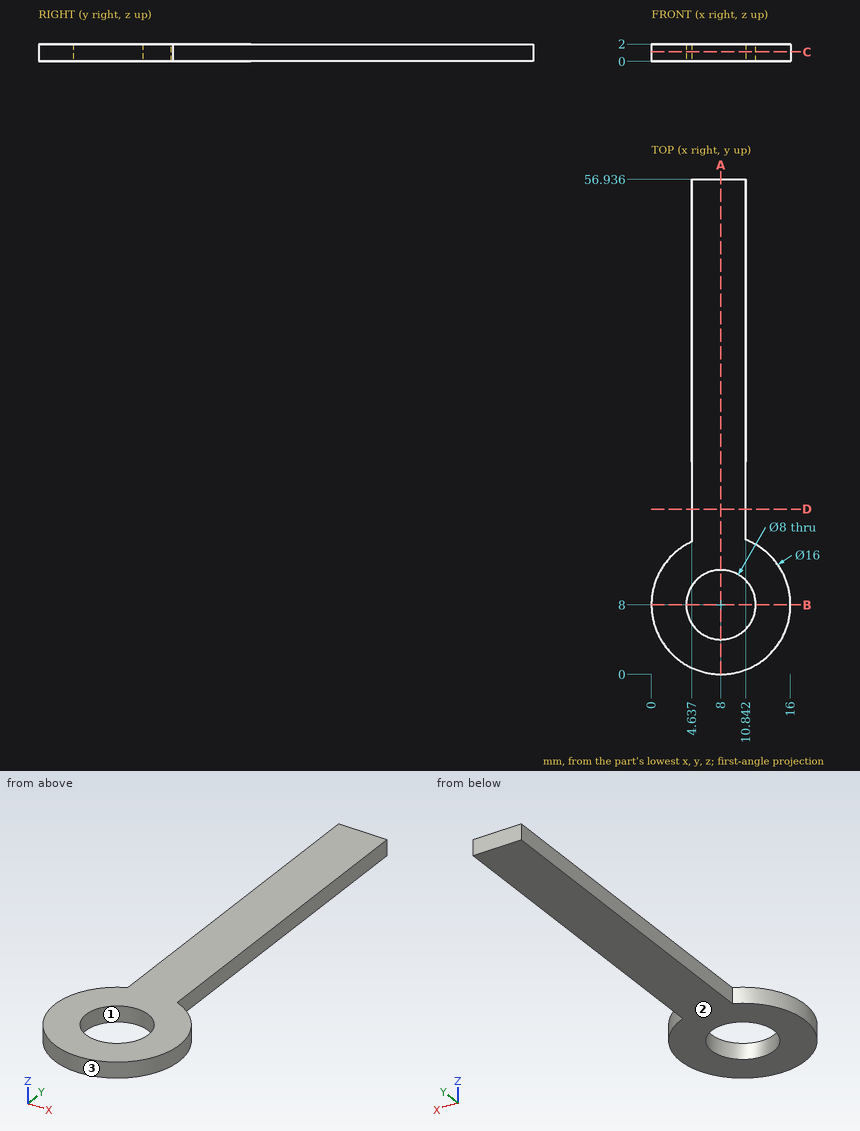
Drawing for the job (mm, zero at the part's lowest x, y, z). Give positions to 0.01 mm unless a question says otherwise; leave off trailing zeros. Order: outer loops, then holes, each group sorted by start corner. A loop starts at its lowest first (then second) coordinate and runs counter-clockwise, first axis right, second up. Notation, with made-up numbers: M 49,30.25 L 105,30.25 A13 cw 105,43.25 Z; hole C 52,-19 d1. An arc over 180 degrees is marked long. Use a Markdown table: item, result. Add a question column.
(1) Saw through at D-D, the plane y = 19. Give the cut face in (x, z).
(2) Drop a flat-ended pin along its axis: P1, Ø0.6, axis at y = 38, z = 1.5, coming from the +X side. Give the stop position or say it passes through.
(3) Saw through at B-B, the plane y = 8. Give the cut face in (x, z).
(4) Mould opens along Y. For the marked faces 1, 2 and 3 say: +Y half, -Y half, draft (parallel to the pull), parting line (faces both ways), or undercut.
(5) Probe line 1 along Y through (x, z) = (8, 1.05) (1 decimal); line 2 along X through (y, z) = (5, 1.3) (1 decimal); line 3 along X through (y, z) = (22, 0.55). List the from-to ranges inside material, lowest first. Write a range as [from, to].
(6) Saw through at C-C, the plane z = 1.1. Give the cut face in (x, y) (1 decimal).
(7) Saw through at A-A, the plane x = 8. Give the cut face in (y, z) (1 decimal).
Answer key:
| question | item | result |
|---|---|---|
| 1 | outline | M 4.64,0 L 10.84,0 L 10.84,2 L 4.64,2 Z |
| 2 | P1 | x = 10.84 |
| 3 | outline | M 0,0 L 4,0 L 4,2 L 0,2 Z; M 12,0 L 16,0 L 16,2 L 12,2 Z |
| 4 | face 1 | undercut |
| 4 | face 2 | draft |
| 4 | face 3 | parting line |
| 5 | line 1 | [0, 4], [12, 56.9] |
| 5 | line 2 | [0.6, 5.4], [10.6, 15.4] |
| 5 | line 3 | [4.64, 10.84] |
| 6 | outline | M 4.6,15.3 A8 ccw long 10.8,15.5 L 10.8,56.9 L 4.6,56.9 Z; hole C 8,8 d8 |
| 7 | outline | M 0,0 L 4,0 L 4,2 L 0,2 Z; M 12,0 L 56.9,0 L 56.9,2 L 12,2 Z |
